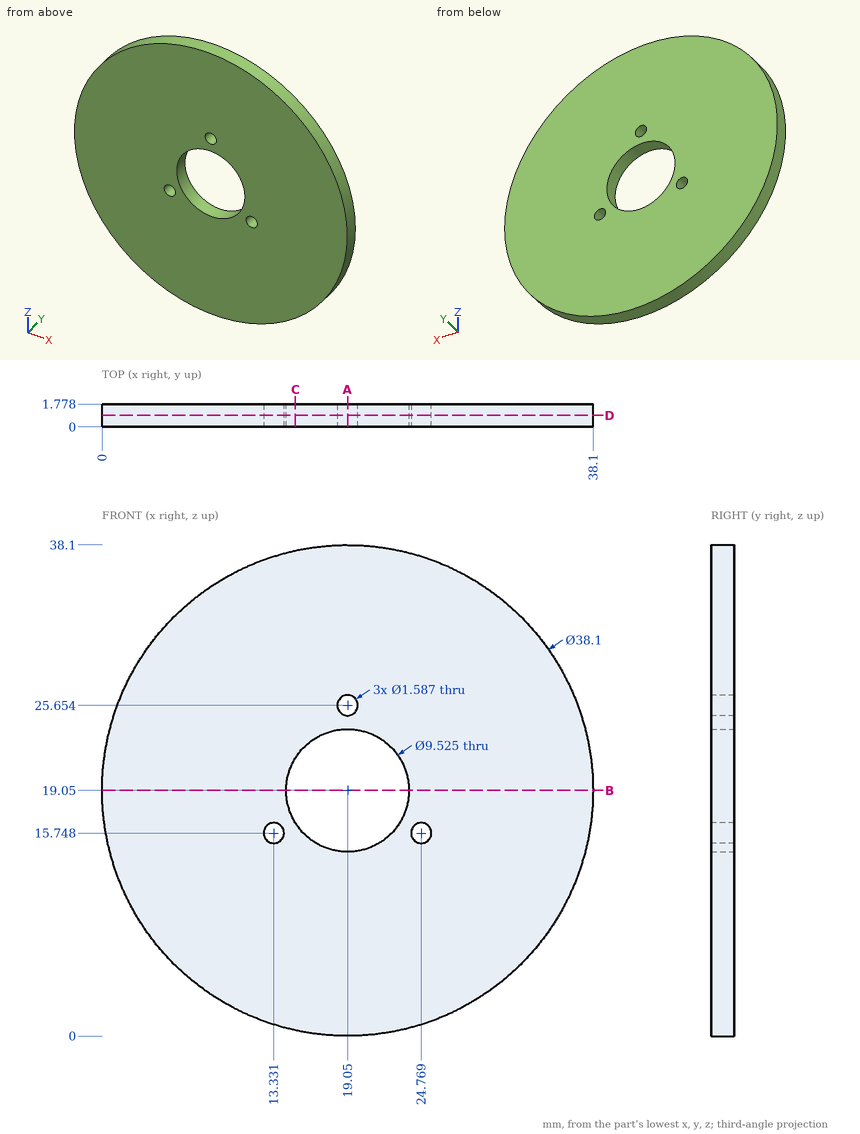
Geometry: see drawing. Coordinates: mm, zero at the bounding-box minimum. Coordinates: 2 decimals unless noted, no trailing zeros. Loops run counter-clockwise (first coordinate to the right, second up) from the corner with the lowest first, then second, coordinate; pieces in that order, holes last. Notation, with made-up numbers: (-13, 50) - (-1, 50) arc R20 ccw to (-1, 71) - close; hole circle Ø7 at (82.5, 88). An arc over 180 degrees is marked (long way). Answer as CSV lines item,"result".
1. Section A-A (x = 19.05). Return loops of the section in (y, z).
Established:
outline,"(0, 0) - (1.78, 0) - (1.78, 14.29) - (0, 14.29) - close; (0, 23.81) - (1.78, 23.81) - (1.78, 24.86) - (0, 24.86) - close; (0, 26.45) - (1.78, 26.45) - (1.78, 38.1) - (0, 38.1) - close"
2. Section B-B (z = 19.05). Return loops of the section in (x, y).
Established:
outline,"(0, 0) - (14.29, 0) - (14.29, 1.78) - (0, 1.78) - close; (23.81, 0) - (38.1, 0) - (38.1, 1.78) - (23.81, 1.78) - close"
3. Contact query for a flat-ended pin moving along its axis: pin 1 (5.5 mm diameter, centred on x = 19.05, z = 19.05, fed in from -Y). Output: stop coordinate, or through.
Established:
pin 1,"passes through"
4. Ray query, line 1 (Z direction, x = 19, y = 1.4); line 2 (X direction, y = 0.9, z = 19.05); line 3 (Z direction, x = 17, y = 0.7). Return the intervals inside material, ascending.
Established:
line 1,"z = 0 to 14.29, 23.81 to 24.86, 26.45 to 38.1"
line 2,"x = 0 to 14.29, 23.81 to 38.1"
line 3,"z = 0.11 to 14.75, 23.35 to 37.99"
5. Section C-C (x = 15). Return loops of the section in (y, z) (1 decimal).
Established:
outline,"(0, 0.4) - (1.8, 0.4) - (1.8, 16.5) - (0, 16.5) - close; (0, 21.6) - (1.8, 21.6) - (1.8, 37.7) - (0, 37.7) - close"
6. Section D-D (y = 0.9). Count the separate pieces of the cut face and the enclosed holes in it, then the cut area to 3 significant figures.
Established:
separate pieces,"1"
enclosed holes,"4"
area,"1,060 mm2"
